```python
from build123d import *

# Parameters (mm, degrees)
BOSS_EXTRUDE1_DEPTH = 1.7272
SKETCH3_R           = 1.05
CUT_EXTRUDE1_DEPTH  = 1.7272


with BuildPart() as part:
    # Sketch1 → Boss-Extrude1 (new body)
    with BuildSketch(Plane.XY):
        Polygon((0, 0), (47.288728977, 29.21), (43.18, 29.21), (43.18, 56.3372), (1.905, 56.3372), (1.905, 29.21), (0, 29.21), (0, 26.7208), (-1.7272, 26.7208), (-1.7272, 24.6888), (0, 24.6888), (0, 6.4008), (-1.7272, 6.4008), (-1.7272, 4.3688), (0, 4.3688), align=None)
        Polygon((2.54, 24.6888), (35.135968928, 24.6888), (2.54, 4.554440863), align=None, mode=Mode.SUBTRACT)
        with BuildLine():
            Line((14.1425, 41.5872), (14.1425, 35.2372))
            Line((14.1425, 35.2372), (30.9425, 35.2372))
            Line((30.9425, 35.2372), (30.9425, 41.5872))
            Line((30.9425, 41.5872), (33.2425, 41.5872))
            ThreePointArc((33.2425, 41.5872), (35.2925, 43.6372), (33.2425, 45.6872))
            Line((33.2425, 45.6872), (30.9425, 45.6872))
            Line((30.9425, 45.6872), (30.9425, 52.0372))
            Line((30.9425, 52.0372), (14.1425, 52.0372))
            Line((14.1425, 52.0372), (14.1425, 45.6872))
            Line((14.1425, 45.6872), (11.8425, 45.6872))
            ThreePointArc((11.8425, 45.6872), (9.7925, 43.6372), (11.8425, 41.5872))
            Line((11.8425, 41.5872), (14.1425, 41.5872))
        make_face(mode=Mode.SUBTRACT)
    extrude(amount=BOSS_EXTRUDE1_DEPTH)

    # Sketch3 → Cut-Extrude1 (cut)
    with BuildSketch(Plane(origin=(22.5425, 43.6372, 1.7272), x_dir=(1, 0, 0), z_dir=(0, 0, 1))):
        with Locations((-18.4568, 10.8495)):
            Circle(SKETCH3_R)
        with Locations((-18.4568, -10.8495)):
            Circle(SKETCH3_R)
        with Locations((18.4568, -10.8495)):
            Circle(SKETCH3_R)
        with Locations((18.4568, 10.8495)):
            Circle(SKETCH3_R)
    extrude(amount=-CUT_EXTRUDE1_DEPTH, mode=Mode.SUBTRACT)


solid = part.part
```
Verification items for the finished model (mm, model axes). A direction names the side the tool comes from. Coordinates: 2 decimals unless noted, no trailing zeros. Loops run counter-clockwise (first coordinate to the right, second up) from the corner with the lowest first, then second, coordinate; pieces in that order, holes last. Notation, with made-up numbers: (81.25, 57.5) - (100.25, 57.5) arc R22 ccw to (100.25, 76.5) - close; hole circle Ø4 at (45, 31.25). An arc over 180 degrees is marked (long way). Answer as a JSON object with one key per item and string values.
(1) Mould release check, pull along Y, two halves, no side actions. Record for faces 1 (the flat face through (13, 45.687, 1)), 2 (the flat face through (23, 56.337, 1)), 3 (the flat face through (0, 28, 1)): pulls with the +Y half, pulls with the -Y half, needs draft (parallel to the pull), parting line crosses it, or undercut.
Response:
{"face 1": "undercut", "face 2": "pulls with the +Y half", "face 3": "needs draft"}
(2) Access from +Z, -Z, +X, -X, +Y, -Y to the whole of each face (thin tool, end or side, straight path). Record for faces 4 (the flat face through (2.54, 14, 1)), 5 (the flat face through (0, 2, 1)), 6 (the flat face through (-1, 26.721, 1)), 7 (the flat face through (-1, 24.689, 1)).
Response:
{"face 4": "+Z, -Z", "face 5": "+Z, -Z, -X, -Y", "face 6": "+Z, -Z, -X, +Y", "face 7": "+Z, -Z, -X"}
(3) Go/stop test with flat-tipped pins: pin 1 Ø1.9 at (x, y) = (4.09, 32.79) entering from -Z; pin 2 Ø0.9 at (x, z) = (46, 1) entering from +Y; pin 3 Ø0.5 at (x, z) = (19.5, 0.5) entering from -Y; pin 4 Ø0.9 at (y, z) = (37.5, 0.5) entering from -X (3 decimals). Record where each tip stops, or that it passes through.
Response:
{"pin 1": "passes through", "pin 2": "stops at y = 29.21", "pin 3": "stops at y = 11.89", "pin 4": "stops at x = 1.905"}
(4) Cross-section at B-B, the plane x = 7. Record the boundary of the cut face in (y, z), then the cut area to 3 significant figures.
Response:
{"outline": "(4.32, 0) - (7.31, 0) - (7.31, 1.73) - (4.32, 1.73) - close; (24.69, 0) - (56.34, 0) - (56.34, 1.73) - (24.69, 1.73) - close", "area": "59.8 mm²"}
(5) Cross-section at A-A, the plane y = 47.5. Record the boundary of the cut face in (x, z) (1 decimal), then the cut area to 3 significant figures.
Response:
{"outline": "(1.9, 0) - (14.1, 0) - (14.1, 1.7) - (1.9, 1.7) - close; (30.9, 0) - (43.2, 0) - (43.2, 1.7) - (30.9, 1.7) - close", "area": "42.3 mm²"}
(6) Cross-section at C-C, the plane x = 16. Record the boundary of the cut face in (y, z).
Response:
{"outline": "(9.88, 0) - (12.87, 0) - (12.87, 1.73) - (9.88, 1.73) - close; (24.69, 0) - (35.24, 0) - (35.24, 1.73) - (24.69, 1.73) - close; (52.04, 0) - (56.34, 0) - (56.34, 1.73) - (52.04, 1.73) - close"}
(7) Scan lines: line 1 along Y through (x, z) = (24, 1.45); line 2 along Y through (x, z) = (31.5, 0.55); line 3 along X through (y, z) = (35.5, 1.4) (1 decimal). Record each from-to range of solid material in increasing order.
Response:
{"line 1": "y = 14.82 to 17.81, 24.69 to 35.24, 52.04 to 56.34", "line 2": "y = 19.46 to 22.44, 24.69 to 41.59, 45.69 to 56.34", "line 3": "x = 1.9 to 14.1, 30.9 to 43.2"}
(8) Cross-section at D-D, the plane z = 1.4. Count the separate pieces of the cut face and the enclosed holes in it, then the cut area to 3 significant figures.
Response:
{"separate pieces": "1", "enclosed holes": "6", "area": "1,160 mm²"}
